from build123d import *

# Parameters (mm, degrees)
SKETCH2_R          = 12.7
CUT_EXTRUDE1_DEPTH = 53


with BuildPart() as part:
    # Sketch1 → Revolve1 (revolve)
    with BuildSketch(Plane.XY, mode=Mode.PRIVATE) as revolve1_sk:
        Polygon((48.64, 0), (48.64, 107.95), (78.615, 107.95), (78.615, 101.6), (136.525, 101.6), (136.525, 63.5), (78.615, 63.5), (57.15, 11.29), (57.15, 0), align=None)
    revolve(revolve1_sk.sketch.rotate(Axis((0, 145.426192893, 0), (0, -1, 0)), 90), axis=Axis((0, 145.426192893, 0), (0, -1, 0)))

    # Sketch2 → Cut-Extrude1 (cut)
    with BuildSketch(Plane(origin=(0, 101.6, 0), x_dir=(1, 0, 0), z_dir=(0, 1, 0))):
        with Locations(Location((-42.17942532, 99.36849893, 0), (0, 0, 270))):
            Circle(SKETCH2_R)
        with Locations(Location((40.438781759, 100.0894971, 0), (0, 0, 270))):
            Circle(SKETCH2_R)
        with Locations(Location((99.36849893, 42.17942532, 0), (0, 0, 270))):
            Circle(SKETCH2_R)
        with Locations(Location((100.0894971, -40.438781759, 0), (0, 0, 270))):
            Circle(SKETCH2_R)
        with Locations(Location((42.17942532, -99.36849893, 0), (0, 0, 270))):
            Circle(SKETCH2_R)
        with Locations(Location((-40.438781759, -100.0894971, 0), (0, 0, 270))):
            Circle(SKETCH2_R)
        with Locations(Location((-99.36849893, -42.17942532, 0), (0, 0, 270))):
            Circle(SKETCH2_R)
        with Locations(Location((-100.0894971, 40.438781759, 0), (0, 0, 270))):
            Circle(SKETCH2_R)
    extrude(amount=-CUT_EXTRUDE1_DEPTH, mode=Mode.SUBTRACT)


solid = part.part
Model file for the job. Use its own axes, mm. A direction names the side the tool comes from. Coordinates: 2 decimals unless noted, no trailing zeros. Loops run counter-clockwise (first coordinate to the right, second up) from the corner with the lowest first, then second, coordinate; pieces in that order, holes last. Notation, with made-up numbers: (0.5, 64.5) -> (49.5, 64.5) arc R27 ccw to (49.5, 97.5) -> close; hole circle Ø9 at (89.5, 18.25). An arc over 180 degrees is marked (long way). Use one line per item in the form item = value. Start each with the question number.
(1) Cut at D-D on y = 91. Give the number of separate pieces and of enclosed holes in the cut face, and give its area (3 significant figures).
(2) Pull direction Z, two halves, no side cores. Call faces 4 (the cylindrical face through (44.254, 82.817, -87.976)), 5 (the flat face through (59, 101.6, -59)), 6 (the cylindrical face through (-41.01, 82.28, 130.22)): pulls with the +Z half, pulls with the -Z half, needs draft (parallel to the pull), parting line crosses it, or undercut.
(3) Cut at B-B on z = 0. Give the cut face in (x, y) (3 decimals), and give its area (3 significant figures).
(4) Cut at A-A on x = 0. Give the cut face in (y, z) (3 decimals).
(5) Tool access for faces 1 (the cylindrical face through (76.746, 104.731, -17.042)), 2 (the flat face through (59, 63.5, 59)), 3 (the cylindrical face through (-111.357, 82.817, -34.579)): list every direction of +Z, -Z, +X, -X, +Y, -Y with a clear straight run to the whole face (end or side of a thin tool).
(6) Probe probe 1 along Z at (x, y) = (-40, 56); probe 2 along X at (y, z) = (51, 8.5); probe 3 along Z at (x, y) = (26.5, 53.5). List the from-to ranges inside material, lowest first. Write a range as from..to.
(7) Flat gauge pins, fed straight in: pin 1 (4 mm diameter, centred on y = 53, z = 51, fed in from -X); pin 2 (5 mm diameter, centred on x = -61, y = 30.5, fed in from +Z); pin 3 (5 mm diameter, centred on x = -27, z = 66.5, fed in from -Y). Where does each tip first touch, or does it go through?
(8) Cut at C-C on x = 106.5. Give the cut face in (y, z).
Values:
q1.separate_pieces = 1
q1.enclosed_holes = 9
q1.area = 47,100 mm2
q2.face_4 = undercut
q2.face_5 = needs draft
q2.face_6 = parting line crosses it
q3.outline = (-136.525, 63.5) -> (-78.615, 63.5) -> (-57.15, 11.29) -> (-57.15, 0) -> (-48.64, 0) -> (-48.64, 107.95) -> (-78.615, 107.95) -> (-78.615, 101.6) -> (-136.525, 101.6) -> close; (48.64, 0) -> (57.15, 0) -> (57.15, 11.29) -> (78.615, 63.5) -> (136.525, 63.5) -> (136.525, 101.6) -> (78.615, 101.6) -> (78.615, 107.95) -> (48.64, 107.95) -> close
q3.area = 9,280 mm2
q4.outline = (0, -57.15) -> (11.29, -57.15) -> (63.5, -78.615) -> (63.5, -136.525) -> (101.6, -136.525) -> (101.6, -78.615) -> (107.95, -78.615) -> (107.95, -48.64) -> (0, -48.64) -> close; (0, 48.64) -> (107.95, 48.64) -> (107.95, 78.615) -> (101.6, 78.615) -> (101.6, 136.525) -> (63.5, 136.525) -> (63.5, 78.615) -> (11.29, 57.15) -> (0, 57.15) -> close
q5.face_1 = +Y
q5.face_2 = -Y
q5.face_3 = +Y, -Y
q6.probe_1 = -64.07..-27.67, 27.67..64.07
q6.probe_2 = -72.98..-47.89, 47.89..72.98
q6.probe_3 = -69.63..-40.79, 40.79..69.63
q7.pin_1 = -56.16
q7.pin_2 = 28.95
q7.pin_3 = 40.78
q8.outline = (63.5, -85.42) -> (101.6, -85.42) -> (101.6, -52.69) -> (63.5, -52.69) -> close; (63.5, -31.67) -> (101.6, -31.67) -> (101.6, 29.48) -> (63.5, 29.48) -> close; (63.5, 51.4) -> (101.6, 51.4) -> (101.6, 85.42) -> (63.5, 85.42) -> close
